from build123d import *

# Parameters (mm, degrees)
EXTRUDE1_DEPTH  = 2.794
HOLE1_D         = 1.60274
EXTRUDE2_DEPTH  = 2.794
LPATTERN1_COUNT = 5
LPATTERN1_PITCH = 2.54
LPATTERN2_COUNT = 63
LPATTERN2_PITCH = 2.54


with BuildPart() as part:
    # Sketch1 → Extrude1 (new body)
    with BuildSketch(Plane(origin=(0, 0, 0), x_dir=(1, 0, 0), z_dir=(0, 1, 0))):
        Polygon((9.854373708, 0.40005), (9.694353708, 0.40005), (9.548747416, 0), (0, 0), (-0.145606292, 0.40005), (-0.305626292, 0.40005), (-0.305626292, 2.13995), (-0.145606292, 2.13995), (0, 2.54), (9.548747416, 2.54), (9.694353708, 2.13995), (9.854373708, 2.13995), align=None)
    extrude(amount=-EXTRUDE1_DEPTH)

    # Hole1 (through all)
    with Locations(Plane(origin=(0.964373708, 0, -1.27), x_dir=(0, 0, 1), z_dir=(0, 1, 0))):
        with Locations((0, 0)):
            hole1 = Hole(HOLE1_D / 2)

    # Sketch4 → Extrude2 (cut)
    with BuildSketch(Plane(origin=(0, 0, 0), x_dir=(1, 0, 0), z_dir=(0, 1, 0))):
        Polygon((1.928772816, 0), (2.5399746, 0), (2.394368308, 0.40005), (2.074379108, 0.40005), align=None)
        Polygon((2.074379108, 2.13995), (2.394368308, 2.13995), (2.5399746, 2.54), (1.928772816, 2.54), align=None)
    extrude2 = extrude(amount=-EXTRUDE2_DEPTH, mode=Mode.SUBTRACT)

    # LPattern1: Hole1 ×5
    with Locations(*[(i * LPATTERN1_PITCH, 0, 0) for i in range(1, LPATTERN1_COUNT)]):
        add(hole1, mode=Mode.SUBTRACT)

    # LPattern2: Extrude2 ×63
    with Locations(*[(i * LPATTERN2_PITCH, 0, 0) for i in range(1, LPATTERN2_COUNT)]):
        add(extrude2, mode=Mode.SUBTRACT)


solid = part.part
Verification items for the finished model (mm, model axes). Round coordinates to 2 decimals unless told otherwise and drop trailing zeros. Order: outer loops, then holes, each group sorted by start corner. A loop starts at its lowest first (then second) coordinate and runs counter-clockwise, first axis right, second up.
1. Release check for a two-part mould opening along X. For faces 1 (the cylindrical face through (5.333, -1.417, -1.64)), 2 (the flat face through (9.854, -1, -1)), 3 (the flat face through (1, -1, -2.54)) record: +X half, -X half, draft (parallel to the pull), parting line (faces both ways), or undercut.
Final values:
face 1: undercut
face 2: +X half
face 3: draft
2. Go/stop test with a flat-tipped pin: P1, Ø1.5, axis at x = 2.5, y = -1, coming from the -Z side. Record where the tip stops, or that it passes through.
Final values:
P1: stops at z = -2.54
3. Section check A-A on z = -1.27. Record the cut outline in (x, y), then the cut area to 3 significant figures.
Final values:
outline: (-0.31, -2.79) - (0.16, -2.79) - (0.16, 0) - (-0.31, 0) - close; (1.77, -2.79) - (2.7, -2.79) - (2.7, 0) - (1.77, 0) - close; (4.31, -2.79) - (5.24, -2.79) - (5.24, 0) - (4.31, 0) - close; (6.85, -2.79) - (7.78, -2.79) - (7.78, 0) - (6.85, 0) - close; (9.39, -2.79) - (9.85, -2.79) - (9.85, 0) - (9.39, 0) - close
area: 10.5 mm2
4. Section check D-D on z = -0.25. Record the cut outline in (x, y), then the cut area to 3 significant figures.
Final values:
outline: (-0.09, -2.79) - (2.02, -2.79) - (2.02, 0) - (-0.09, 0) - close; (2.45, -2.79) - (4.56, -2.79) - (4.56, 0) - (2.45, 0) - close; (4.99, -2.79) - (7.1, -2.79) - (7.1, 0) - (4.99, 0) - close; (7.53, -2.79) - (9.64, -2.79) - (9.64, 0) - (7.53, 0) - close
area: 23.6 mm2
5. Section check B-B on x = 8. Record the cut outline in (y, z).
Final values:
outline: (-2.79, -2.54) - (0, -2.54) - (0, -1.82) - (-2.79, -1.82) - close; (-2.79, -0.72) - (0, -0.72) - (0, 0) - (-2.79, 0) - close
6. Section check C-C on z = -2.4. Record the cut outline in (x, y), then the cut area to 3 significant figures.
Final values:
outline: (-0.05, -2.79) - (1.98, -2.79) - (1.98, 0) - (-0.05, 0) - close; (2.49, -2.79) - (4.52, -2.79) - (4.52, 0) - (2.49, 0) - close; (5.03, -2.79) - (7.06, -2.79) - (7.06, 0) - (5.03, 0) - close; (7.57, -2.79) - (9.6, -2.79) - (9.6, 0) - (7.57, 0) - close
area: 22.7 mm2
7. Thickness scan on L1, parallel to X at y = -1, z = -1.27; L2, parallel to X at y = -1.25, z = -1.4; L3, parallel to X at y = -1.9, z = -0.2. Record the ranges inside material, lowest first.
Final values:
L1: x = -0.31 to 0.16, 1.77 to 2.7, 4.31 to 5.24, 6.85 to 7.78, 9.39 to 9.85
L2: x = -0.31 to 0.17, 1.76 to 2.71, 4.3 to 5.25, 6.84 to 7.79, 9.38 to 9.85
L3: x = -0.07 to 2, 2.47 to 4.54, 5.01 to 7.08, 7.55 to 9.62
